from build123d import *

# Parameters (mm, degrees)
SKETCH1_W           = 82
SKETCH1_H           = 240
BOSS_EXTRUDE1_DEPTH = 18
CUT_EXTRUDE1_DEPTH  = 19
FILLET1_R           = 7


with BuildPart() as part:
    # Sketch1 → Boss-Extrude1 (new body)
    with BuildSketch(Plane.XY):
        with Locations((41, 120)):
            Rectangle(SKETCH1_W, SKETCH1_H)
    extrude(amount=BOSS_EXTRUDE1_DEPTH)

    # Sketch2 → Cut-Extrude1 (cut, through all)
    with BuildSketch(Plane.XY):
        with BuildLine():
            Line((39.251228148, 59.5), (42.748771852, 59.5))
            ThreePointArc((42.748771852, 59.5), (43.339438857, 59.400327171), (43.864690916, 59.11234721))
            ThreePointArc((43.864690916, 59.11234721), (50.5, 59.5), (50.88765279, 66.135309084))
            ThreePointArc((50.88765279, 66.135309084), (50.599672829, 66.660561143), (50.5, 67.251228148))
            Line((50.5, 67.251228148), (50.5, 172.748771852))
            ThreePointArc((50.5, 172.748771852), (50.599672829, 173.339438857), (50.88765279, 173.864690916))
            ThreePointArc((50.88765279, 173.864690916), (50.5, 180.5), (43.864690916, 180.88765279))
            ThreePointArc((43.864690916, 180.88765279), (43.339438857, 180.599672829), (42.748771852, 180.5))
            Line((42.748771852, 180.5), (39.251228148, 180.5))
            ThreePointArc((39.251228148, 180.5), (38.660561143, 180.599672829), (38.135309084, 180.88765279))
            ThreePointArc((38.135309084, 180.88765279), (31.5, 180.5), (31.11234721, 173.864690916))
            ThreePointArc((31.11234721, 173.864690916), (31.400327171, 173.339438857), (31.5, 172.748771852))
            Line((31.5, 172.748771852), (31.5, 67.251228148))
            ThreePointArc((31.5, 67.251228148), (31.400327171, 66.660561143), (31.11234721, 66.135309084))
            ThreePointArc((31.11234721, 66.135309084), (31.5, 59.5), (38.135309084, 59.11234721))
            ThreePointArc((38.135309084, 59.11234721), (38.660561143, 59.400327171), (39.251228148, 59.5))
        make_face()
    extrude(amount=CUT_EXTRUDE1_DEPTH, mode=Mode.SUBTRACT)

    # Fillet1
    fillet1_edges = [part.edges().sort_by_distance(p)[0] for p in [
        (0, 240, 9),
        (82, 240, 9),
        (82, 0, 9),
        (0, 0, 9),
    ]]
    fillet(fillet1_edges, radius=FILLET1_R)


solid = part.part
Part model, mm, in its own coordinate system. A direction names the side the tool comes from. Give positions to 0.01 mm unless a question says otherwise; leave off trailing zeros. Loops run counter-clockwise (first coordinate to the right, second up) from the corner with the lowest first, then second, coordinate; pieces in that order, holes last.
(1) Pull direction X, two halves, no side cores. Call faces 3 (the flat face through (31, 122, 0)), 4 (the cylindrical face through (31.4, 59.6, 8.9)), 5 (the cylindrical face through (79.9, 238, 9.1)): pulls with the +X half, pulls with the -X half, needs draft (parallel to the pull), parting line crosses it, or undercut.
Return value:
face 3: needs draft
face 4: undercut
face 5: pulls with the +X half
(2) Band-saw the part on B-B (z = 12.5). Write the cut outline in (x, y), and give its area (3 significant figures).
Return value:
outline: (0, 7) arc R7 ccw to (7, 0) - (75, 0) arc R7 ccw to (82, 7) - (82, 233) arc R7 ccw to (75, 240) - (7, 240) arc R7 ccw to (0, 233) - close; hole (31.11, 66.14) arc R5 ccw to (38.14, 59.11) arc R1.8 cw to (39.25, 59.5) - (42.75, 59.5) arc R1.8 cw to (43.86, 59.11) arc R5 ccw to (50.89, 66.14) arc R1.8 cw to (50.5, 67.25) - (50.5, 172.75) arc R1.8 cw to (50.89, 173.86) arc R5 ccw to (43.86, 180.89) arc R1.8 cw to (42.75, 180.5) - (39.25, 180.5) arc R1.8 cw to (38.14, 180.89) arc R5 ccw to (31.11, 173.86) arc R1.8 cw to (31.5, 172.75) - (31.5, 67.25) arc R1.8 cw to start
area: 17,300 mm2
(3) Drill centre lines: line 1 along X through (y, z) = (130, 1.75); line 2 along Y through (x, z) = (40, 9); line 3 along Y through (x, z) = (35.5, 5.75). Where is each one in solid material? Low to high.
Return value:
line 1: x = 0 to 31.5, 50.5 to 82
line 2: y = 0 to 59.5, 180.5 to 240
line 3: y = 0 to 58.06, 181.94 to 240
(4) Band-saw the part on A-A (y = 77.5). Write the cut outline in (x, z), and give its area (3 significant figures).
Return value:
outline: (0, 0) - (31.5, 0) - (31.5, 18) - (0, 18) - close; (50.5, 0) - (82, 0) - (82, 18) - (50.5, 18) - close
area: 1,130 mm2
(5) 3-axis set-ups, long thin cutter, end or side, ignore diameter. For faces 1 (the flat face through (31.5, 121, 9)), 2 (the cylindrical face through (79.9, 2, 9.1)): which of +Z, -Z, +X, -X, +Y, -Y reach the whole face in a straight line?
Return value:
face 1: +Z, -Z
face 2: +Z, -Z, +X, -Y
